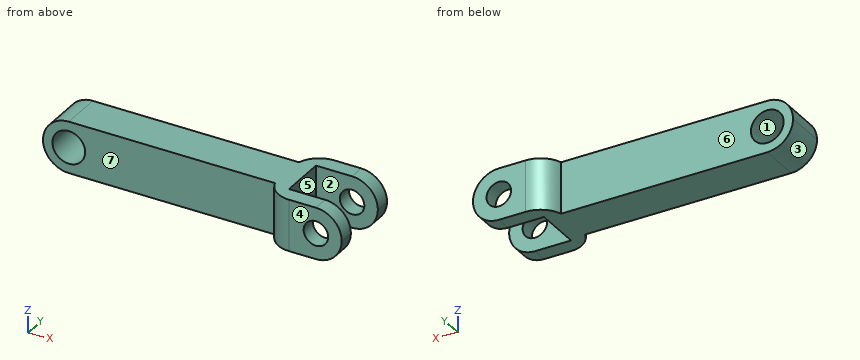
```python
from build123d import *

# Parameters (mm, degrees)
SKETCH1_W           = 60
SKETCH1_H           = 15
BOSS_EXTRUDE1_DEPTH = 10
SKETCH2_W           = 12
SKETCH2_H           = 8.9375
CUT_EXTRUDE1_DEPTH  = 63.649820431
SKETCH4_W           = 45
SKETCH4_H           = 3.53125
CUT_EXTRUDE3_DEPTH  = 63.649820431
FILLET1_R           = 5
FILLET2_R           = 5
SKETCH3_R           = 3.175
SKETCH3_R_2         = 2.38125
CUT_EXTRUDE2_DEPTH  = 63.649820431


# Some blends are built 0.0001 mm under size
with BuildPart() as part:
    # Sketch1 → Boss-Extrude1 (new body)
    with BuildSketch(Plane.XY):
        with Locations((30, 7.5)):
            Rectangle(SKETCH1_W, SKETCH1_H)
    extrude(amount=BOSS_EXTRUDE1_DEPTH)

    # Sketch2 → Cut-Extrude1 (cut, through all)
    with BuildSketch(Plane.XY.offset(10)):
        with Locations((54, 7.5)):
            Rectangle(SKETCH2_W, SKETCH2_H)
    extrude(amount=-CUT_EXTRUDE1_DEPTH, mode=Mode.SUBTRACT)

    # Sketch4 → Cut-Extrude3 (cut, through all)
    with BuildSketch(Plane.XY.offset(10)):
        with Locations((22.5, 13.234375)):
            Rectangle(SKETCH4_W, SKETCH4_H)
        with Locations((22.5, 1.765625)):
            Rectangle(SKETCH4_W, SKETCH4_H)
    extrude(amount=-CUT_EXTRUDE3_DEPTH, mode=Mode.SUBTRACT)

    # Fillet1
    fillet1_edges = [part.edges().sort_by_distance(p)[0] for p in [
        (60, 1.515625, 0),
        (60, 1.515625, 10),
        (60, 13.484375, 0),
        (60, 13.484375, 10),
        (0, 7.5, 0),
        (0, 7.5, 10),
    ]]
    fillet(fillet1_edges, radius=FILLET1_R - 0.0001)  # a hair under: the kernel refuses the full size

    # Fillet2
    # the kernel refuses this fillet: 5 mm, written as the material it takes off along each edge
    with BuildSketch(Plane(origin=(45, 0, 21.948528528), x_dir=(1, 0, 0), z_dir=(0, 0, -1))) as fillet2_piece_1:
        with BuildLine():
            CenterArc((4.779411411, -5), FILLET2_R, 90, 72.917402966)
            Line((0, -3.53125), (-0.095588228, -3.501875))
            ThreePointArc((-0.095588228, -3.501875), (-0.1, -1.765625), (-0.1, 0))
            Line((-0.1, 0), (0, 0.1))
            Line((0, 0.1), (4.779411411, 0.1))
            Line((4.779411411, 0.1), (4.779411411, 0))
        make_face()
    extrude(amount=33.897057056, mode=Mode.SUBTRACT)
    with BuildSketch(Plane(origin=(45, 15, 21.948528528), x_dir=(0, -1, 0), z_dir=(0, 0, -1))) as fillet2_piece_2:
        with BuildLine():
            CenterArc((5, -4.779411411), FILLET2_R, 107.082597034, 72.917402966)
            Line((0, -4.779411411), (-0.1, -4.779411411))
            Line((-0.1, -4.779411411), (-0.1, 0))
            Line((-0.1, 0), (0, 0.1))
            ThreePointArc((0, 0.1), (1.765625, 0.1), (3.501875, 0.095588228))
            Line((3.501875, 0.095588228), (3.53125, 0))
        make_face()
    extrude(amount=33.897057056, mode=Mode.SUBTRACT)

    # Sketch3 → Cut-Extrude2 (cut, through all)
    with BuildSketch(Plane(origin=(0, 15, 0), x_dir=(1, 0, 0), z_dir=(0, 1, 0))):
        with Locations(Location((5, -5, 0), (0, 0, 270))):
            Circle(SKETCH3_R)
        with Locations(Location((55, -5, 0), (0, 0, 270))):
            Circle(SKETCH3_R_2)
    extrude(amount=-CUT_EXTRUDE2_DEPTH, mode=Mode.SUBTRACT)


solid = part.part
```
Work out the finished part from the listing and answer in its coordinate system (mm). Face numbers are marked on the shaded views. A direction names the side the tool comes from. Coordinates: 2 decimals unless noted, no trailing zeros. Loops run counter-clockwise (first coordinate to the right, second up) from the corner with the lowest first, then second, coordinate; pieces in that order, holes last. Notation, with made-up numbers: M 25.5,82.5 L 50.5,82.5 A17 cw 50.5,106.5 Z; hole C 55,76.5 d2. An arc over 180 degrees is marked long. Use CSV: the item, a comma, the result in double quotes. Start each with the question number.
(1) For a pull along Z with two mould halves and no side action, classify the marked faces 1, 2 and 3 as +Z half, -Z half, draft (parallel to the pull), parting line (faces both ways), or undercut.
(2) Find section A-A, the plane z = 3.5. Give the vertices of the cut face in (x, y), then the cut area to 3 significant figures.
(3) Find section C-C, the plane x = 14.5. Give the vertices of the cut face in (y, z), then the cut area to 3 significant figures.
(4) For the marked faces 4, 5, 6 and 7, determine the directions among +Z, -Z, +X, -X, +Y, -Y from which every point of the face is accessible in a straight line to the end or side of a thin tool.
(5) Given pin 1 Ø4.5 at (y, z) = (5.5, 5.5) entering from +X; pin 2 Ø4 at (x, z) = (11.5, 7) entering from -Y; pin 3 Ø1 at (x, z) = (17, 6) entering from +Y, each flat-ended and moving along its own axis, determine where each tip first touches the part or whether it passes through.
(6) Consider line 1 (Y direction, x = 51.5, z = 6); line 2 (Y direction, x = 32, z = 3.25); line 3 (Z direction, x = 6.5, y = 4.5). Determine where each line is inside the solid, lowest interval first.
Recorded:
1,face 1,"undercut"
1,face 2,"draft"
1,face 3,"-Z half"
2,outline,"M 0.23,3.53 L 2.2,3.53 L 2.2,11.47 L 0.23,11.47 Z; M 7.8,3.53 L 45,3.53 A5 ccw 49.78,0 L 53.15,0 L 53.15,3.03 L 48,3.03 L 48,11.97 L 53.15,11.97 L 53.15,15 L 49.78,15 A5 ccw 45,11.47 L 7.8,11.47 Z; M 56.85,0 L 59.77,0 L 59.77,3.03 L 56.85,3.03 Z; M 56.85,11.97 L 59.77,11.97 L 59.77,15 L 56.85,15 Z"
2,area,"396 mm^2"
3,outline,"M 3.53,0 L 11.47,0 L 11.47,10 L 3.53,10 Z"
3,area,"79.4 mm^2"
4,face 4,"+Z, -Z, +X, -X, -Y"
4,face 5,"+Z, -Z, +X"
4,face 6,"+Z, -Z, -X, +Y"
4,face 7,"+Z, -Z, -X, -Y"
5,pin 1,"stops at x = 48"
5,pin 2,"stops at y = 3.53"
5,pin 3,"stops at y = 11.47"
6,line 1,"y = 0 to 3.03, 11.97 to 15"
6,line 2,"y = 3.53 to 11.47"
6,line 3,"z = 0 to 2.2, 7.8 to 10"
